Geometry check sheet. Reference: drawing and pictorial views, mm from the part's lowest x, y, z. Coordinates: 2 decimals unless noted, no trailing zeros. Loops run counter-clockwise (first coordinate to the right, second up) from the corner with the lowest first, then second, coordinate; pieces in that order, holes last. Notation, with made-up numbers: (87, 22.25) -> (126, 22.25) arc R33 cw to (126, 57.25) -> close; hole circle Ø1 at (20, 7.25). An arc over 180 degrees is marked (long way). Answer as a JSON object with one key per item and string values.
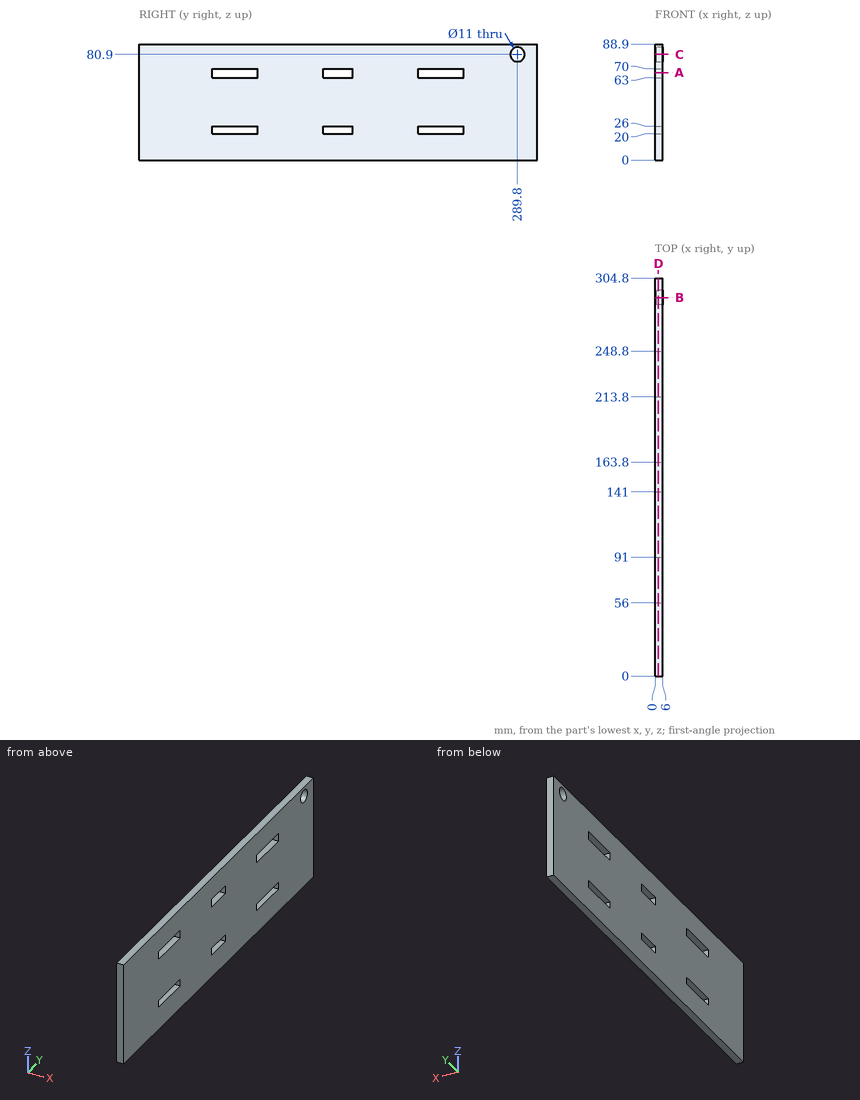
1. Section check D-D, the plane x = 2.45. State how many separate pieces and enclosed holes the cut face has, then the cut area to 3 significant figures.
Evaluation:
{"separate pieces": "1", "enclosed holes": "7", "area": "25,800 mm^2"}
2. Section check A-A, the plane z = 67. Record the boundary of the cut face in (x, y), then the cut area to 3 significant figures.
Evaluation:
{"outline": "(0, 0) -> (6, 0) -> (6, 56) -> (0, 56) -> close; (0, 91) -> (6, 91) -> (6, 141) -> (0, 141) -> close; (0, 163.8) -> (6, 163.8) -> (6, 213.8) -> (0, 213.8) -> close; (0, 248.8) -> (6, 248.8) -> (6, 304.8) -> (0, 304.8) -> close", "area": "1,270 mm^2"}
3. Section check B-B, the plane y = 289.8. Record the boundary of the cut face in (x, z).
Evaluation:
{"outline": "(0, 0) -> (6, 0) -> (6, 75.4) -> (0, 75.4) -> close; (0, 86.4) -> (6, 86.4) -> (6, 88.9) -> (0, 88.9) -> close"}
4. Thickness scan on probe 1 along Y at (x, z) = (4.55, 68.5); probe 2 along Z at (x, y) = (4.2, 65); probe 3 along Y at (x, z) = (3.75, 80.9). Record the ranges inside material, lowest first. Write a range as from..to.
Evaluation:
{"probe 1": "y = 0..56, 91..141, 163.8..213.8, 248.8..304.8", "probe 2": "z = 0..20, 26..63, 70..88.9", "probe 3": "y = 0..284.3, 295.3..304.8"}
5. Section check C-C, the plane z = 80.9. Record the boundary of the cut face in (x, y), then the cut area to 3 significant figures.
Evaluation:
{"outline": "(0, 0) -> (6, 0) -> (6, 284.3) -> (0, 284.3) -> close; (0, 295.3) -> (6, 295.3) -> (6, 304.8) -> (0, 304.8) -> close", "area": "1,760 mm^2"}
